For this review, take the finished solid that the model builds, in its own axes (mm). A direction names the side the tool comes from. Give positions to 0.01 mm unless a question says otherwise; leave off trailing zeros. Loops run counter-clockwise (first coordinate to the right, second up) from the corner with the lowest first, then second, coordinate; pieces in that order, holes last. Notation, with made-up numbers: (76.25, 26) - (134.25, 26) arc R17 cw to (134.25, 59) - close; hole circle Ø2 at (6, 31). An arc over 180 degrees is marked (long way). Answer in a Markdown table with one row per item.
Autodesk Inventor part; units mm, degrees
ref_plane "YZ Plane" through (0, 0, 0) normal (1, 0, 0) x (0, 1, 0)
ref_plane "XZ Plane" through (0, 0, 0) normal (0, 1, 0) x (-1, 0, 0)
ref_plane "XY Plane" through (0, 0, 0) normal (0, 0, 1) x (1, 0, 0)
sketch "Эскиз1" plane through (0, 0, 0) normal (0, 0, 1) x (1, 0, 0)
  line L0 (-6.8, -1.5588) -> (-9.5, -3.1177)
  line L1 (-9.5, -3.1177) -> (-12.2, -1.5588)
  circle A0 centre (-9.5, 0) radius 1.5
  line L2 (-6.8, 1.5588) -> (-6.8, -1.5588)
  line L3 (-12.2, -1.5588) -> (-12.2, 1.5588)
  line L4 (-9.5, 3.1177) -> (-6.8, 1.5588)
  line L5 (-12.2, 1.5588) -> (-9.5, 3.1177)
  line L6 (6.8, -1.5588) -> (6.8, 1.5588)
  line L7 (6.8, 1.5588) -> (9.5, 3.1177)
  line L8 (9.5, -3.1177) -> (6.8, -1.5588)
  circle A1 centre (9.5, 0) radius 1.5
  line L9 (9.5, 3.1177) -> (12.2, 1.5588)
  line L10 (12.2, 1.5588) -> (12.2, -1.5588)
  line L11 (12.2, -1.5588) -> (9.5, -3.1177)
  line L12 (-12.2, 5) -> (12.2, 5)
  line L13 (14.2, 3) -> (14.2, -3)
  line L14 (12.2, -5) -> (-12.2, -5)
  line L15 (-14.2, -3) -> (-14.2, 3)
  arc A2 (-12.2, 5) -> (-14.2, 3) centre (-12.2, 3) ccw
  arc A3 (-14.2, -3) -> (-12.2, -5) centre (-12.2, -3) ccw
  arc A4 (12.2, -5) -> (14.2, -3) centre (12.2, -3) ccw
  arc A5 (14.2, 3) -> (12.2, 5) centre (12.2, 3) ccw
  line L16 (0, 0) -> (0, 2.3671) construction
  point P0 (14.2, 0)
  point P1 (-14.2, 0)
  point P2 (0, 5)
  dimension "Width" = 10
  dimension "d6" = 2
  dimension "d12" = 13.6
extrude "Выдавливание1" add sketch "Эскиз1" against normal blind 1.5 contours L0 L1 L3 L5 L4 L2 | L6 L7 L9 L10 L11 L8 | L12 A5 L13 A4 L14 A3 L15 A2
extrude "Выдавливание2" add sketch "Эскиз1" along normal blind 2.5 contours L12 A5 L13 A4 L14 A3 L15 A2
chamfer "Фаска1" distance 0.3 distance2 0.1 8 edges at (0, 5, -1.5) (13.6142, 4.4142, -1.5) (14.2, 0, -1.5) (13.6142, -4.4142, -1.5) (0, -5, -1.5) (-13.6142, -4.4142, -1.5) (-14.2, 0, -1.5) (-13.6142, 4.4142, -1.5) measured on face at (2.8826, -3.7448, -1.5)
equation "\"d8\" = Thick - Nut_thick"
equation "\"Thick\" = 4"
properties part number "Крепежи динамиков"
1. Wall thickness on line 1 (X direction, y = -0.75, z = 1.25); line 2 (Y direction, x = -9.5, z = -1.1); line 3 (Y direction, x = -12, z = 0.95): over which ranges is each line inside the solid? List them lowest first. Write a range as [from, to].
Values:
| item | result |
|---|---|
| line 1 | x = [-14.2, -12.2], [-6.8, 6.8], [12.2, 14.2] |
| line 2 | y = [-5, -1.5], [1.5, 5] |
| line 3 | y = [-5, -1.67], [1.67, 5] |
2. For faces 4 (the face through (13.6, 4.43, 0.52)), 5 (the face through (-10.869, 2.327, 1.232)), list the 3-axis set-ups (+Z, -Z, +X, -X, +Y, -Y) from which the entire face can be reached by the end or side of a thin tool; tool diameter is ignored.
Values:
| item | result |
|---|---|
| face 4 | +Z, -Z, +X, +Y |
| face 5 | +Z |
3. We need section D-D, the plane z = 2.25. Give the boundary of the cut face in (x, y), and give its area (3 significant figures).
Values:
| item | result |
|---|---|
| outline | (-14.2, -3) arc R2 ccw to (-12.2, -5) - (12.2, -5) arc R2 ccw to (14.2, -3) - (14.2, 3) arc R2 ccw to (12.2, 5) - (-12.2, 5) arc R2 ccw to (-14.2, 3) - close; hole (-12.2, -1.56) - (-9.5, -3.12) - (-6.8, -1.56) - (-6.8, 1.56) - (-9.5, 3.12) - (-12.2, 1.56) - close; hole (6.8, -1.56) - (9.5, -3.12) - (12.2, -1.56) - (12.2, 1.56) - (9.5, 3.12) - (6.8, 1.56) - close |
| area | 230 mm^2 |
4. We need section A-A, the plane y = 0. Give the boundary of the cut face in (x, z).
Values:
| item | result |
|---|---|
| outline | (-14.2, -1.4) - (-13.9, -1.5) - (-11, -1.5) - (-11, 0) - (-12.2, 0) - (-12.2, 2.5) - (-14.2, 2.5) - close; (-8, -1.5) - (8, -1.5) - (8, 0) - (6.8, 0) - (6.8, 2.5) - (-6.8, 2.5) - (-6.8, 0) - (-8, 0) - close; (11, -1.5) - (13.9, -1.5) - (14.2, -1.4) - (14.2, 2.5) - (12.2, 2.5) - (12.2, 0) - (11, 0) - close |
5. Mouldability with a two-part tool opening along X and no side actions: class faces 1 (the face through (0, 0, 2.5)), 2 (the face through (6.8, 0, 1)), 3 (the face through (-13.52, -4.3, -1.45)) as released by +X, released by -X, zero draft, split by the parting line, or undercut.
Values:
| item | result |
|---|---|
| face 1 | zero draft |
| face 2 | undercut |
| face 3 | released by -X |
6. We need section C-C, the plane y = -2.25. Give the boundary of the cut face in (x, z).
Values:
| item | result |
|---|---|
| outline | (-14.2, -1.4) - (-13.9, -1.5) - (13.9, -1.5) - (14.2, -1.4) - (14.2, 2.5) - (11, 2.5) - (11, 0) - (8, 0) - (8, 2.5) - (-8, 2.5) - (-8, 0) - (-11, 0) - (-11, 2.5) - (-14.2, 2.5) - close |
7. We need section B-B, the plane z = -1.1. Give the boundary of the cut face in (x, y).
Values:
| item | result |
|---|---|
| outline | (-14.2, -3) arc R2 ccw to (-12.2, -5) - (12.2, -5) arc R2 ccw to (14.2, -3) - (14.2, 3) arc R2 ccw to (12.2, 5) - (-12.2, 5) arc R2 ccw to (-14.2, 3) - close; hole circle Ø3 at (-9.5, 0); hole circle Ø3 at (9.5, 0) |
